Verification items for the finished model (mm, model axes). Coordinates: 2 decimals unless noted, no trailing zeros. Order: outer loops, then holes, each group sorted by start corner. A loop starts at its lowest first (then second) coordinate and runs counter-clockwise, first axis right, second up. Notation, with made-up numbers: M -34.5,11 L 3.5,11 A25 ccw 3.5,49 Z; hole C 75,49 d1. An arc over 180 degrees is marked long. Answer as a JSON object with one key per item and string values. Group by question number.
(1) Mould release check, pull along Y, two halves, no side actions. Record for faces 1 (the face through (2.1, 48.64, 5.99)), 2 (the face through (2.16, 2.1, 5.99)), 3 (the face through (16.71, 27.546, 3.131)): released by +Y, released by -Y, zero draft, split by the parting line, or undercut.
(2) Cross-section at C-C (y = 25.4). Enter the section's corners in (x, z) (3 decimals), plus the area to 3 significant figures.
(3) Cross-section at B-B (x = 19.05). Enter the section's corners in (y, z) (3 decimals).
(4) Cross-section at A-A (z = 1.75). Enter the section's corners in (x, y) (3 decimals).
(5) Cross-section at D-D (z = 5.75). Enter the section's corners in (x, y) (3 decimals), plus the area to 3 significant figures.
(6) Material ranges on line 1 (Y direction, x = 19.05, z = 4) (3 decimals); line 2 (X direction, y = 23, z = 5.25); line 3 (X direction, y = 28, z = 1), recorded low to high.
from build123d import *

# Parameters (mm, degrees)
F0_W     = 38.1
F0_H     = 50.8
F0_R     = 3.175
F1_DEPTH = 6.35
F2_R     = 5.08
F3_SIZE  = 1.27


with BuildPart() as f1:
    # F0 (on Top) → F1 (new body)
    with BuildSketch(Plane.XY):
        with Locations((19.05, 25.4)):
            Rectangle(F0_W, F0_H)
        with Locations((19.05, 25.4)):
            Circle(F0_R, mode=Mode.SUBTRACT)
    extrude(amount=F1_DEPTH)

    # F2
    f2_edges = [f1.edges().sort_by_distance(p)[0] for p in [
        (0, 50.8, 3.175),
        (0, 0, 3.175),
        (38.1, 0, 3.175),
        (38.1, 50.8, 3.175),
    ]]
    fillet(f2_edges, radius=F2_R)

    # F3
    f3_edges = [f1.edges().sort_by_distance(p)[0] for p in [
        (19.05, 50.8, 6.35),
    ]]
    chamfer(f3_edges, length=F3_SIZE)


solid = f1.part
Taken from the geometry:
{
 "1": {"face 1": "released by +Y", "face 2": "released by -Y", "face 3": "undercut"},
 "2": {"outline": "M 0,0 L 15.875,0 L 15.875,6.35 L 1.27,6.35 L 0,5.08 Z; M 22.225,0 L 38.1,0 L 38.1,5.08 L 36.83,6.35 L 22.225,6.35 Z", "area": "200 mm²"},
 "3": {"outline": "M 0,0 L 22.225,0 L 22.225,6.35 L 1.27,6.35 L 0,5.08 Z; M 28.575,0 L 50.8,0 L 50.8,5.08 L 49.53,6.35 L 28.575,6.35 Z"},
 "4": {"outline": "M 0,5.08 A5.08 ccw 5.08,0 L 33.02,0 A5.08 ccw 38.1,5.08 L 38.1,45.72 A5.08 ccw 33.02,50.8 L 5.08,50.8 A5.08 ccw 0,45.72 Z; hole C 19.05,25.4 d6.35"},
 "5": {"outline": "M 0.67,5.08 A4.41 ccw 5.08,0.67 L 33.02,0.67 A4.41 ccw 37.43,5.08 L 37.43,45.72 A4.41 ccw 33.02,50.13 L 5.08,50.13 A4.41 ccw 0.67,45.72 Z; hole C 19.05,25.4 d6.35", "area": "1,770 mm²"},
 "6": {"line 1": "y = 0 to 22.225, 28.575 to 50.8", "line 2": "x = 0.17 to 16.97, 21.13 to 37.93", "line 3": "x = 0 to 17.23, 20.87 to 38.1"}
}
